from build123d import *

# Parameters (mm, degrees)
F1_DEPTH  = 30
F2_W      = 133
F2_H      = 3
F3_DEPTH  = 5
F5_DEPTH  = 16.501
F6_R      = 13
F7_W      = 146.5
F7_H      = 30
F8_DEPTH  = 4.5
F10_DEPTH = 2
F11_W     = 9
F11_H     = 60
F12_DEPTH = 2.001


with BuildPart() as f1:
    # F0 (on Top) → F1 (new body)
    with BuildSketch(Plane.XY):
        Polygon((-51.263781, 32.674184), (-48.263781, -2.628919), (-48.263781, 37.371081), (-30.263781, 37.371081), (-30.263781, -112.628919), (102.736219, -112.628919), (102.736219, -109.628919), (-27.263781, -109.628919), (-27.263781, 40.371081), (-51.263781, 40.371081), align=None)
    extrude(amount=F1_DEPTH)

    # F2 (on face) → F3 (join)
    with BuildSketch(Plane.XZ.offset(112.628919)):
        with Locations((36.236219, 15)):
            Rectangle(F2_W, F2_H)
    extrude(amount=F3_DEPTH)

    # F4 (on face) → F5 (cut, through all)
    with BuildSketch(Plane.XY.offset(16.5)):
        Polygon((102.736219, -112.628919), (-30.263781, -117.628919), (102.736219, -117.628919), align=None)
    extrude(amount=-F5_DEPTH, mode=Mode.SUBTRACT)

    # F6
    f6_edges = [f1.edges().sort_by_distance(p)[0] for p in [
        (102.736219, -111.128919, 0),
        (102.736219, -111.128919, 30),
    ]]
    fillet(f6_edges, radius=F6_R)

    # F7 (on face) → F8 (join)
    with BuildSketch(Plane.YZ.offset(-27.263781)):
        with Locations((-32.878919, 15)):
            Rectangle(F7_W, F7_H)
    extrude(amount=F8_DEPTH)

    # F9 (on face) → F10 (join)
    with BuildSketch(Plane.XY.offset(30)):
        Polygon((89.736219, -109.628919), (-22.763781, 40.371081), (-22.763781, -106.128919), (-27.263781, -106.128919), (-27.263781, -109.628919), align=None)
    extrude(amount=-F10_DEPTH)

    # F11 (on face) → F12 (cut, through all)
    with BuildSketch(Plane(origin=(0, 0, 28), x_dir=(1, 0, 0), z_dir=(0, 0, -1))):
        with Locations((-18.263781, 76.128919)):
            Rectangle(F11_W, F11_H)
    extrude(amount=-F12_DEPTH, mode=Mode.SUBTRACT)


solid = f1.part
Model file for the job. Use its own axes, mm. A direction names the side the tool comes from. Round coordinates to 2 decimals unless told otherwise and drop trailing zeros. Order: outer loops, then holes, each group sorted by start corner. A loop starts at its lowest first (then second) coordinate and runs counter-clockwise, first axis right, second up.
(1) Band-saw the part on D-D (x = 68). List the corners of the cut face in (y, z).
(2) Band-saw the part on B-B (x = -16). List the corners of the cut face in (y, z), then the cut area to 3 significant figures.
(3) Drill centre lines: line 1 (X direction, y = -5, z = 13); line 2 (Z direction, x = -10, y = 12.5); line 3 (Y direction, x = -35, z = 9.75). Where is each one in solid material? Low to high.
(4) Band-saw the part on C-C (z = 19). List the corners of the cut face in (x, y).
(5) Pull direction Y, two halves, no side cores. Call faces 1 (the face through (-25, -106.129, 14)), 2 (the face through (-39, 37.371, 15)), 3 (the face through (21, -115, 16.5)): released by +Y, released by -Y, zero draft, split by the parting line, or undercut.
(6) 3-axis set-ups, long thin cutter, end or side, ignore diameter. For faces 4 (the face through (35, -112.629, 23)), 5 (the face through (-48.264, 17, 15)), 6 (the face through (21, -115, 13.5)), 7 (the face through (-27.264, -108, 14)): which of +Z, -Z, +X, -X, +Y, -Y reach the whole face in a straight line?
(7) Pin check, flat tips, straight feed: pin 1 (8 mm diameter, centred on y = 8.5, z = 27, fed in from +X); pin 2 (12 mm diameter, centred on x = 71, z = 19.5, fed in from +Y); pin 3 (0.6 mm diameter, centred on y = -68.5, z = 28.5, fed in from -X); pin 4 (10 mm diameter, centred on x = 63.5, y = -58.5, fed in from -Z). Stop position of each tip, or through.
(8) Band-saw the part on A-A (y = 16.5). List the corners of the cut face in (x, z).
Verdict:
1. outline: (-113.93, 13.5) - (-112.63, 13.5) - (-112.63, 0) - (-109.63, 0) - (-109.63, 28) - (-80.65, 28) - (-80.65, 30) - (-112.63, 30) - (-112.63, 16.5) - (-113.93, 16.5) - close
2. outline: (-117.09, 13.5) - (-112.63, 13.5) - (-112.63, 0) - (-109.63, 0) - (-109.63, 28) - (-106.13, 28) - (-106.13, 30) - (-112.63, 30) - (-112.63, 16.5) - (-117.09, 16.5) - close; (-46.13, 28) - (31.35, 28) - (31.35, 30) - (-46.13, 30) - close
2. area: 265 mm2
3. line 1: x = -30.26 to -22.76
3. line 2: z = 28 to 30
3. line 3: y = 37.37 to 40.37
4. outline: (-51.26, 32.67) - (-48.26, -2.63) - (-48.26, 37.37) - (-30.26, 37.37) - (-30.26, -112.63) - (102.58, -112.63) - (102.58, -109.63) - (-27.26, -109.63) - (-27.26, -106.13) - (-22.76, -106.13) - (-22.76, 40.37) - (-51.26, 40.37) - close
5. face 1: undercut
5. face 2: released by -Y
5. face 3: zero draft
6. face 4: +Z, +X, -X, -Y
6. face 5: +Z, -Z, -Y
6. face 6: -Z, +X, -X, -Y
6. face 7: -Z, +X
7. pin 1: stops at x = 4.04
7. pin 2: stops at y = -109.63
7. pin 3: stops at x = -30.26
7. pin 4: passes through
8. outline: (-49.89, 0) - (-48.26, 0) - (-48.26, 30) - (-49.89, 30) - close; (-30.26, 0) - (-22.76, 0) - (-22.76, 28) - (-4.86, 28) - (-4.86, 30) - (-30.26, 30) - close
